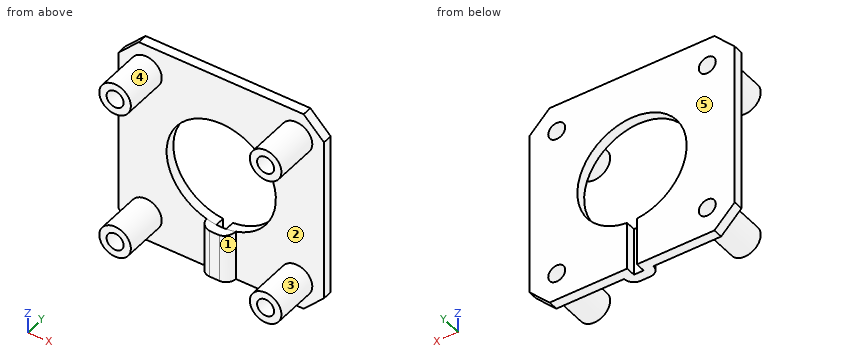
```python
from build123d import *
from build123d.topology import SkipClean

# Parameters (mm, degrees)
SKETCH1_R               = 3.25
BOSS_EXTRUDE1_DEPTH     = 11.15
SKETCH2_W               = 42.3
SKETCH2_H               = 42.3
SKETCH2_R               = 11.25
BOSS_EXTRUDE2_DEPTH     = 2
CUT_EXTRUDE1_DEPTH      = 32.921270338
SKETCH4_R               = 1.75
CUT_EXTRUDE2_DEPTH      = 32.921270338
MIRROR6_COPY_1_SKETCH_R = 1.75
MIRROR6_COPY_1_DEPTH    = 32.921270338
BOSS_EXTRUDE3_DEPTH     = 2
CUT_EXTRUDE3_DEPTH      = 2
FILLET1_R               = 2


with BuildPart() as part:
    # Sketch1 → Boss-Extrude1 (new body)
    with BuildSketch(Plane(origin=(0, 0, 0), x_dir=(1, 0, 0), z_dir=(0, 1, 0))):
        with Locations(Location((-15.5, 15.5, 0), (0, 0, 270))):
            Circle(SKETCH1_R)
    extrude(amount=BOSS_EXTRUDE1_DEPTH)


with BuildPart() as body_2:
    # Mirror2: mirrored copy
    add(part.part.mirror(Plane(origin=(0, 0, 0), x_dir=(0, 0, 1), z_dir=(1, 0, 0))))


with BuildPart() as body_3:
    # Mirror3: mirrored copy
    add(part.part.mirror(Plane.XY))


with BuildPart() as body_4:
    # Mirror3 2: mirrored copy
    add(body_2.part.mirror(Plane.XY))


with BuildPart() as part_1:
    add(part.part)

    add(body_2.part)  # Boss-Extrude2 merges body 2

    add(body_3.part)  # Boss-Extrude2 merges body 3

    add(body_4.part)  # Boss-Extrude2 merges body 4
    # Sketch2 → Boss-Extrude2 (add)
    with BuildSketch(Plane(origin=(0, 11.15, 0), x_dir=(1, 0, 0), z_dir=(0, 1, 0))):
        Rectangle(SKETCH2_W, SKETCH2_H)
        with Locations(Location((0, 0, 0), (0, 0, 270))):
            Circle(SKETCH2_R, mode=Mode.SUBTRACT)
    extrude(amount=-BOSS_EXTRUDE2_DEPTH)

    # Sketch3 → Cut-Extrude1 (cut, through all)
    with BuildSketch(Plane(origin=(0, 11.15, 0), x_dir=(1, 0, 0), z_dir=(0, 1, 0))):
        Polygon((-16.963055506, 21.15), (-21.15, 16.963055506), (-21.15, 21.15), align=None)
        Polygon((16.963055506, -21.15), (21.15, -16.963055506), (21.15, -21.15), align=None)
    cut_extrude1 = extrude(amount=-CUT_EXTRUDE1_DEPTH, mode=Mode.SUBTRACT)

    # Mirror4: Cut-Extrude1 across plane
    add(cut_extrude1.mirror(Plane.XY), mode=Mode.SUBTRACT)

    # Sketch4 → Cut-Extrude2 (cut, through all)
    with BuildSketch(Plane.XZ):
        with Locations(Location((15.5, -15.5, 0), (0, 0, 270))):
            Circle(SKETCH4_R)
    cut_extrude2 = extrude(amount=-CUT_EXTRUDE2_DEPTH, mode=Mode.SUBTRACT)

    # Mirror5: Cut-Extrude2 across plane
    add(cut_extrude2.mirror(Plane(origin=(0, 0, 0), x_dir=(0, 0, 1), z_dir=(1, 0, 0))), mode=Mode.SUBTRACT)

    # Mirror6: Cut-Extrude2 across plane
    add(cut_extrude2.mirror(Plane.XY), mode=Mode.SUBTRACT)

    # Mirror6 copy 1 sketch → Mirror6 copy 1 (cut, through all)
    with BuildSketch(Plane(origin=(0, 0, 0), x_dir=(-1, 0, 0), z_dir=(0, -1, 0))):
        with Locations(Location((15.5, -15.5, 0), (0, 0, 270))):
            Circle(MIRROR6_COPY_1_SKETCH_R)
    extrude(amount=-MIRROR6_COPY_1_DEPTH, mode=Mode.SUBTRACT)

    # Sketch6 → Boss-Extrude3 (add)
    with SkipClean():  # the faces are left unmerged after this step: merging them gives an invalid solid
        with BuildSketch(Plane.XZ.offset(-9.15)):
            with BuildLine():
                Line((-3, -21.15), (-3, -10.842624221))
                ThreePointArc((-3, -10.842624221), (0, -11.25), (3, -10.842624221))
                Line((3, -10.842624221), (3, -21.15))
                Line((3, -21.15), (-3, -21.15))
            make_face()
        extrude(amount=BOSS_EXTRUDE3_DEPTH)

    # Sketch7 → Cut-Extrude3 (cut)
    with SkipClean():  # the faces are left unmerged after this step: merging them gives an invalid solid
        with BuildSketch(Plane(origin=(0, 11.15, 0), x_dir=(1, 0, 0), z_dir=(0, 1, 0))):
            with BuildLine():
                Line((-1, 11.25), (-1, 21.15))
                ThreePointArc((-1, 21.15), (0, 22.15), (1, 21.15))
                Line((1, 21.15), (1, 11.25))
                ThreePointArc((1, 11.25), (0, 10.25), (-1, 11.25))
            make_face()
        extrude(amount=-CUT_EXTRUDE3_DEPTH, mode=Mode.SUBTRACT)

    # Fillet1
    fillet1_edges = [part_1.edges().sort_by_distance(p)[0] for p in [
        (3, 7.15, -15.996312111),
        (-3, 7.15, -15.996312111),
    ]]
    fillet(fillet1_edges, radius=FILLET1_R - 0.0001)  # a hair under: the kernel refuses the full size


solid = part_1.part
```
Work out the finished part from the listing and answer in its coordinate system (mm). Face numbers are marked on the shaded views. A direction names the side the tool comes from. Round coordinates to 2 decimals unless told otherwise and drop trailing zeros. Loops run counter-clockwise (first coordinate to the right, second up) from the corner with the lowest first, then second, coordinate; pieces in that order, holes last.
(1) Each of these flat-tipped pins is pushed along its axis until it touches: P1, Ø3, axis at x = -15.5, z = -15.5, coming from the +Y side; P2, Ø1, axis at x = 0, z = -14.5, coming from the +Y side; P3, Ø8, axis at x = 11.5, z = -4, coming from the -Y side; P4, Ø1.6, axis at x = -0.5, z = -17.5, coming from the -Y side. Where does it stop, or does it pass through?
Computed values:
P1: passes through
P2: stops at y = 9.15
P3: stops at y = 9.15
P4: stops at y = 7.15
(2) Find the intervals of material crossed by L1, parallel to Z at x = -15.5, y = 9.25; L2, parallel to X at y = 5, z = -15.5; L3, parallel to X at y = 7.75, z = -15.5, in increasing order.
Computed values:
L1: z = -21.15 to -17.25, -13.75 to 13.75, 17.25 to 21.15
L2: x = -18.75 to -17.25, -13.75 to -12.25, 12.25 to 13.75, 17.25 to 18.75
L3: x = -18.75 to -17.25, -13.75 to -12.25, -2.43 to 2.43, 12.25 to 13.75, 17.25 to 18.75
(3) The part is cut by section C-C, the plane z = 9. Give the vertices of the cut face in (x, y).
Computed values:
outline: (-21.15, 9.15) - (-6.75, 9.15) - (-6.75, 11.15) - (-21.15, 11.15) - close; (6.75, 9.15) - (21.15, 9.15) - (21.15, 11.15) - (6.75, 11.15) - close
(4) The part is cut by section A-A, the plane y = 3.5. Give the vertices of the cut face in (x, z), and give its area (3 significant figures).
Computed values:
outline: circle Ø6.5 at (-15.5, -15.5); circle Ø6.5 at (-15.5, 15.5); circle Ø6.5 at (15.5, -15.5); circle Ø6.5 at (15.5, 15.5); hole circle Ø3.5 at (-15.5, -15.5); hole circle Ø3.5 at (-15.5, 15.5); hole circle Ø3.5 at (15.5, -15.5); hole circle Ø3.5 at (15.5, 15.5)
area: 94.2 mm2
(5) The part is cut by section B-B, the plane z = -15.5. Give the number of separate pieces and of enclosed holes in the cut face, and give its area (3 significant figures).
Computed values:
separate pieces: 3
enclosed holes: 0
area: 132 mm2
(6) The mould has two halves that part along X. Classify the marked faces 3, 4 and 5: pulls with the +X half, pulls with the -X half, needs draft (parallel to the pull), parting line crosses it, or undercut.
Computed values:
face 3: undercut
face 4: undercut
face 5: needs draft
(7) The part is cut by section D-D, the plane x = -15.5. Give the vertices of the cut face in (y, z), and give its area (4 significant figures).
Computed values:
outline: (0, -18.75) - (9.15, -18.75) - (9.15, -21.15) - (11.15, -21.15) - (11.15, -17.25) - (0, -17.25) - close; (0, -13.75) - (11.15, -13.75) - (11.15, 13.75) - (0, 13.75) - (0, 12.25) - (9.15, 12.25) - (9.15, -12.25) - (0, -12.25) - close; (0, 17.25) - (11.15, 17.25) - (11.15, 21.15) - (9.15, 21.15) - (9.15, 18.75) - (0, 18.75) - close
area: 125.5 mm2
(8) For the marked faces 1 and 2, determine the directions among +Z, -Z, +X, -X, +Y, -Y from which every point of the face is accessible in a straight line to the end or side of a thin tool.
Computed values:
face 1: +Z, -Z, -Y
face 2: -Y
